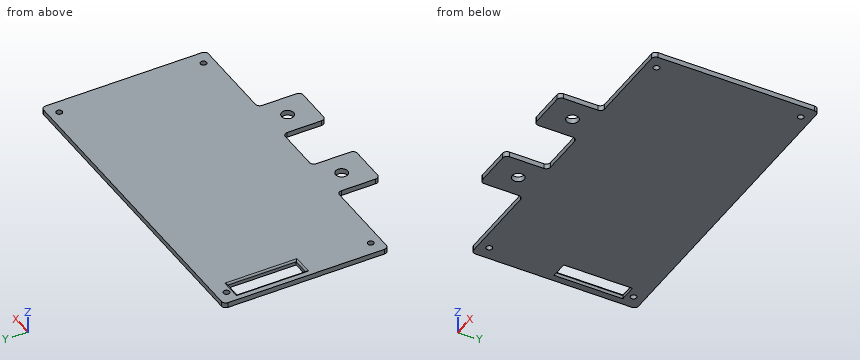
```python
from build123d import *

# Parameters (mm, degrees)
SKETCH020_R   = 3.5
SKETCH020_R_2 = 1.75
SKETCH020_W   = 10
SKETCH020_H   = 40
PAD012_DEPTH  = 3
FILLET008_R   = 2.5
FILLET009_R   = 1


with BuildPart() as part:
    # Sketch020 → Pad012 (new body)
    with BuildSketch(Plane.XY):
        Polygon((-94.5, 48), (-94.5, -48), (-41, -48), (-41, -73), (-15, -73), (-15, -48), (15, -48), (15, -73), (41, -73), (41, -48), (94.5, -48), (94.5, 48), align=None)
        with Locations((-28, -58)):
            Circle(SKETCH020_R, mode=Mode.SUBTRACT)
        with Locations((28, -58)):
            Circle(SKETCH020_R, mode=Mode.SUBTRACT)
        with Locations((-86.5, -42)):
            Circle(SKETCH020_R_2, mode=Mode.SUBTRACT)
        with Locations((86.5, -42)):
            Circle(SKETCH020_R_2, mode=Mode.SUBTRACT)
        with Locations((86.5, 42)):
            Circle(SKETCH020_R_2, mode=Mode.SUBTRACT)
        with Locations((-86.5, 42)):
            Circle(SKETCH020_R_2, mode=Mode.SUBTRACT)
        with Locations((-85.5, 18)):
            Rectangle(SKETCH020_W, SKETCH020_H, mode=Mode.SUBTRACT)
    extrude(amount=PAD012_DEPTH)

    # Fillet008
    fillet008_edges = [part.edges().sort_by_distance(p)[0] for p in [
        (94.5, -48, 1.5),
        (41, -48, 1.5),
        (41, -73, 1.5),
        (94.5, 48, 1.5),
        (15, -48, 1.5),
        (15, -73, 1.5),
        (-15, -48, 1.5),
        (-15, -73, 1.5),
        (-41, -73, 1.5),
        (-41, -48, 1.5),
        (-94.5, -48, 1.5),
        (-94.5, 48, 1.5),
    ]]
    fillet(fillet008_edges, radius=FILLET008_R)

    # Fillet009
    fillet009_edges = [part.edges().sort_by_distance(p)[0] for p in [
        (-90.5, 18, 3),
        (-85.5, 38, 3),
        (-80.5, 18, 3),
        (-85.5, -2, 3),
    ]]
    fillet(fillet009_edges, radius=FILLET009_R)


with BuildPart() as part_1:
    # Body008 placement: moved
    add(part.part.moved(Location((0, 87, 2.5))))


solid = part_1.part
```
The model under review builds one solid part; all positions refer to its coordinate system, in mm. Round coordinates to 2 decimals unless told otherwise and drop trailing zeros. Loops run counter-clockwise (first coordinate to the right, second up) from the corner with the lowest first, then second, coordinate; pieces in that order, holes last. Notation, with made-up numbers: M 6,4.25 L 13,4.25 A24 cw 13,30.25 Z; hole C -9.75,-1.75 d10. An arc over 180 degrees is marked long. Put each result on its own line as item: value.
Q1. Consider section B-B, the plane y = 88. Give the boundary of the cut face in (x, z), then the cut area to 3 significant figures.
Result set:
outline: M -94.5,2.5 L -90.5,2.5 L -90.5,4.5 A1 ccw -91.5,5.5 L -94.5,5.5 Z; M -80.5,2.5 L 94.5,2.5 L 94.5,5.5 L -79.5,5.5 A1 ccw -80.5,4.5 Z
area: 537 mm²
Q2. For pin 1 (4 mm diameter, centred on x = 86.5, y = 45, fed in from -Z); pin 2 (1.5 mm diameter, centred on x = -58, z = 4, fed in from -Y); pin 3 (0.9 mm diameter, centred on y = 27.5, z = 4, fed in from +X); pin 4 (1.5 mm diameter, centred on y = 28.5, z = 3.5, fed in from -X), all flat-tipped, find the tip position at first contact; note any pin that passes through.
Result set:
pin 1: stops at z = 2.5
pin 2: stops at y = 39
pin 3: stops at x = 41
pin 4: stops at x = -41
Q3. To check wall thickness, follow L1, parallel to Y at x = -86.5, z = 4.55; L2, parallel to X at y = 129, z = 3.8; L3, parallel to Y at x = 86.5, z = 3.7. State the ranges of each line that lie inside material, in increasing order.
Result set:
L1: y = 39 to 43.25, 46.75 to 85, 125 to 127.25, 130.75 to 135
L2: x = -94.5 to -88.25, -84.75 to 84.75, 88.25 to 94.5
L3: y = 39 to 43.25, 46.75 to 127.25, 130.75 to 135
Q4. Consider section C-C, the plane z = 3.25. Count the separate pieces of the cut face and the enclosed holes in it, then the cut area to 3 significant figures.
Result set:
separate pieces: 1
enclosed holes: 7
area: 18,900 mm²
Q5. Consider section A-A, the plane x = -28. Give the boundary of the cut face in (y, z), then the cut area to 3 significant figures.
Result set:
outline: M 14,2.5 L 25.5,2.5 L 25.5,5.5 L 14,5.5 Z; M 32.5,2.5 L 135,2.5 L 135,5.5 L 32.5,5.5 Z
area: 342 mm²
Q6. Consider section D-D, the plane x = 49. Give the boundary of the cut face in (y, z), then the cut area to 3 significant figures.
Result set:
outline: M 39,2.5 L 135,2.5 L 135,5.5 L 39,5.5 Z
area: 288 mm²
